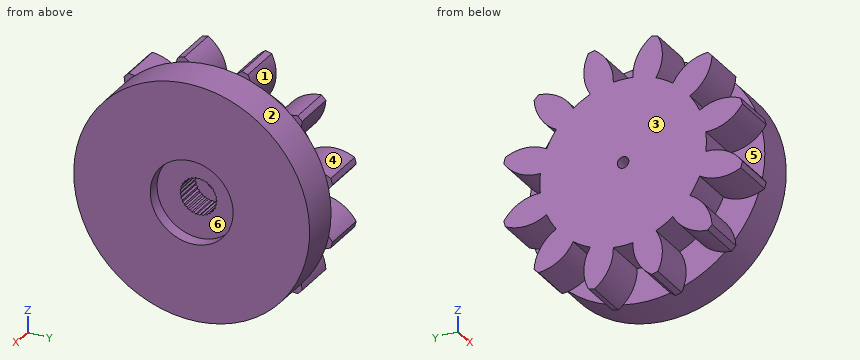
```python
from build123d import *

# Parameters (mm, degrees)
BASPROSKE_W         = 7
BASPROSKE_H         = 19.25
TOOTHCUT_DEPTH      = 29.109162207
TEETHCUTS_COUNT     = 12
TEETHCUTS_ANGLE     = 330
BORSKE_R            = 0.4
BORE_DEPTH          = 50.0000508
EXTRUDE_START       = 6.3
SKETCH_1_R          = 18.5
SKETCH_1_R_2        = 0.4
EXTRUDE_1_DEPTH     = 6.3
SKETCH_8_R          = 6.5
SKETCH_8_R_2        = 0.4
CUT_EXTRUDE_6_DEPTH = 2
SKETCH_9_R          = 0.4
CUT_EXTRUDE_7_DEPTH = 4.4
SKETCH_10_R         = 0.9
CUT_EXTRUDE_8_DEPTH = 30.621500794


with BuildPart() as part:
    # BasProSke → Base-Revolve (revolve)
    with BuildSketch(Plane(origin=(0, 0, 0), x_dir=(1, 0, 0), z_dir=(0, 1, 0)), mode=Mode.PRIVATE) as base_revolve_sk:
        with Locations((3.5, 9.625)):
            Rectangle(BASPROSKE_W, BASPROSKE_H)
    revolve(base_revolve_sk.sketch.rotate(Axis((-10, 0, 0), (1, 0, 0)), 180), axis=Axis((-10, 0, 0), (1, 0, 0)))

    # TooCutSke → ToothCut (cut, through all)
    with BuildSketch(Plane(origin=(0, 0, 0), x_dir=(0, 0, -1), z_dir=(1, 0, 0))):
        with BuildLine():
            ThreePointArc((1.535617211, 12.970916006), (0, 13.0615), (-1.535617211, 12.970916006))
            ThreePointArc((-1.535617211, 12.970916006), (-2.27635986, 16.247221969), (-4.533719407, 18.734631928))
            ThreePointArc((-4.533719407, 18.734631928), (0, 19.2754), (4.533719407, 18.734631928))
            ThreePointArc((4.533719407, 18.734631928), (2.27635986, 16.247221969), (1.535617211, 12.970916006))
        make_face()
    toothcut = extrude(amount=TOOTHCUT_DEPTH, mode=Mode.SUBTRACT)

    # TeethCuts: ToothCut ×12 about axis
    teethcuts_axis = Axis((-10, 0, 0), (1, 0, 0))
    for i in range(1, TEETHCUTS_COUNT):
        add(toothcut.rotate(teethcuts_axis, i * TEETHCUTS_ANGLE / (TEETHCUTS_COUNT - 1)), mode=Mode.SUBTRACT)

    # BorSke → Bore (cut, symmetric)
    with BuildSketch(Plane(origin=(0, 0, 0), x_dir=(0, 0, -1), z_dir=(1, 0, 0))):
        with Locations(Location((0, 0, 0), (0, 0, 180))):
            Circle(BORSKE_R)
    extrude(amount=BORE_DEPTH, both=True, mode=Mode.SUBTRACT)

    # Эскиз1 → Бобышка-Вытянуть1 (add)
    with BuildSketch(Plane(origin=(7, 0, 0), x_dir=(0, 0, -1), z_dir=(1, 0, 0)).offset(EXTRUDE_START)):
        with Locations(Location((0, 0, 0), (0, 0, 168.366396173))):
            Circle(SKETCH_1_R)
        Circle(SKETCH_1_R_2, mode=Mode.SUBTRACT)
    extrude(amount=-EXTRUDE_1_DEPTH)

    # Эскиз8 → Вырез-Вытянуть6 (cut)
    with BuildSketch(Plane(origin=(13.3, 0, 0), x_dir=(0, 0, -1), z_dir=(1, 0, 0))):
        Circle(SKETCH_8_R)
        Circle(SKETCH_8_R_2, mode=Mode.SUBTRACT)
    extrude(amount=-CUT_EXTRUDE_6_DEPTH, mode=Mode.SUBTRACT)

    # Эскиз9 → Вырез-Вытянуть7 (cut)
    with BuildSketch(Plane(origin=(11.3, 0, 0), x_dir=(0, 0, -1), z_dir=(1, 0, 0))):
        Polygon((0.297449416, 2.735002218), (0, 2.9), (-0.297449416, 2.735002218), (-0.623414277, 2.832199612), (-0.878439845, 2.607116554), (-1.217678395, 2.631968717), (-1.418355403, 2.357325017), (-1.755005224, 2.308669891), (-1.891950238, 1.997307583), (-2.21026996, 1.877420226), (-2.277079583, 1.543898266), (-2.562184929, 1.358384478), (-2.555735218, 1.018297982), (-2.794294978, 0.775832182), (-2.714887514, 0.445083216), (-2.8957469, 0.157002835), (-2.747094688, -0.148943146), (-2.861796915, -0.46916779), (-2.650850767, -0.736005093), (-2.694032487, -1.07340065), (-2.43065601, -1.288652259), (-2.400298095, -1.62744249), (-2.09680648, -1.781043478), (-1.994328431, -2.105386927), (-1.66491261, -2.190155083), (-1.495106186, -2.484885811), (-1.155169276, -2.496857471), (-0.925974437, -2.748194196), (-0.59141151, -2.686809578), (-0.313545153, -2.883000076), (0, -2.751129456), (0.313545153, -2.883000076), (0.59141151, -2.686809578), (0.925974437, -2.748194196), (1.155169276, -2.496857471), (1.495106186, -2.484885811), (1.66491261, -2.190155083), (1.994328431, -2.105386927), (2.09680648, -1.781043478), (2.400298095, -1.62744249), (2.43065601, -1.288652259), (2.694032487, -1.07340065), (2.650850767, -0.736005093), (2.861796915, -0.46916779), (2.747094688, -0.148943146), (2.8957469, 0.157002835), (2.714887514, 0.445083216), (2.794294978, 0.775832182), (2.555735218, 1.018297982), (2.562184929, 1.358384478), (2.277079583, 1.543898266), (2.21026996, 1.877420226), (1.891950238, 1.997307583), (1.755005224, 2.308669891), (1.418355403, 2.357325017), (1.217678395, 2.631968717), (0.878439845, 2.607116554), (0.623414277, 2.832199612), align=None)
        Circle(SKETCH_9_R, mode=Mode.SUBTRACT)
    extrude(amount=-CUT_EXTRUDE_7_DEPTH, mode=Mode.SUBTRACT)

    # Эскиз10 → Вырез-Вытянуть8 (cut, through all)
    with BuildSketch(Plane.ZY):
        Circle(SKETCH_10_R)
    extrude(amount=-CUT_EXTRUDE_8_DEPTH, mode=Mode.SUBTRACT)


solid = part.part
```
Geometry: final body of the model. Coordinates: model frame, mm. Face numbers are marked on the shaded views. A direction names the side the tool comes from. Coordinates: 2 decimals unless noted, no trailing zeros. Write each loop counter-clockwise with the first axis right and the second up, starting at its lowest first coordinate (ties: lowest second). Pieces come first, ordered by that corner, then holes. Notation, with made-up numbers: M -15.75,-34 L -8.75,-34 A13 cw -8.75,-12 Z; hole C -17.5,89 d7. An arc over 180 degrees is marked long. Answer as CSV lines item,"result". Start each with the question number.
Q1. Cut plane A-A on z = -15.5. Return the cut outline in (x, y), then the cut area to 3 significant figures.
Q2. Pin query (flat end, axial travel): P1, Ø0.9, axis at y = 18, z = -5, coming from the +X side; P2, Ø1.5, axis at x = 8.5, y = -6.5, coming from the -Z side; P3, Ø2, axis at x = 10.5, y = 1.5, coming from the -Z side; P4, Ø3.5, axis at y = -9, z = 15, coming from the -X side. Return the tip coordinate at first contact, or that it passes through.
Q3. Mould query, pull axis Y, two halves, no side actions, for the marked faces 1, 2 and 3. Classes: released by +Y, released by -Y, zero draft, split by the parting line, or undercut.
Q4. Reachability of the marked faces 4, 5 and 6 from +Z, -Z, +X, -X, +Y, -Y: full face, straight path, thin tool, end or side. Return the list, or none.
Q5. Line query: line 1 (Y direction, x = 12.7, z = 0); line 2 (Y direction, x = 5, z = -11). Output: solid intervals per line, ascending. Write a range as from..to.
Q6. Cut plane B-B on z = 14.5. Return the cut outline in (x, y), then the cut area to 3 significant figures.
Findings below:
1,outline,"M 0,-6.16 L 7,-6.16 L 7,-10.1 L 13.3,-10.1 L 13.3,10.1 L 7,10.1 L 7,6.16 L 0,6.16 L 0,1.94 L 7,1.94 L 7,-1.94 L 0,-1.94 Z"
1,area,"186 mm2"
2,P1,"stops at x = 13.3"
2,P2,"stops at z = -17.58"
2,P3,"stops at z = -18.49"
2,P4,"stops at x = 7"
3,face 1,"undercut"
3,face 2,"split by the parting line"
3,face 3,"zero draft"
4,face 4,"-X"
4,face 5,"-X, -Y"
4,face 6,"+X"
5,line 1,"y = -18.5..-6.5, 6.5..18.5"
5,line 2,"y = -13.41..-8.13, -7.04..7.04, 8.13..13.41"
6,outline,"M 0,-6.08 L 7,-6.08 L 7,-11.49 L 13.3,-11.49 L 13.3,11.49 L 7,11.49 L 7,6.08 L 0,6.08 L 0,1.66 L 7,1.66 L 7,-1.66 L 0,-1.66 Z"
6,area,"207 mm2"
